Verification items for the finished model (mm, model axes). A direction names the side the tool comes from. Give positions to 0.01 mm unless a question says otherwise; leave off trailing zeros. Write each loop counter-clockwise with the first axis right and the second up, starting at its lowest first coordinate (ties: lowest second). Pieces come first, ordered by that corner, then holes. Notation, with made-up numbers: M 51,-23.75 L 67,-23.75 A20 ccw 67,14.25 Z; hole C 56,66.5 d6. An arc over 180 degrees is marked long. Answer as a JSON object with one key per item and string values.
```python
from build123d import *

# Parameters (mm, degrees)
CROQUIS1_W              = 100
CROQUIS1_H              = 100
SALIENTE_EXTRUIR1_DEPTH = 5
CHAFL_N1_SIZE2          = 2.886751346
CHAFL_N1_SIZE           = 5
CORTAR_EXTRUIR1_REACH   = 72.887
CROQUIS2_W              = 25
CROQUIS2_H              = 35


with BuildPart() as part:
    # Croquis1 → Saliente-Extruir1 (new body)
    with BuildSketch(Plane(origin=(0, 0, 0), x_dir=(1, 0, 0), z_dir=(0, 1, 0))):
        Rectangle(CROQUIS1_W, CROQUIS1_H)
    extrude(amount=SALIENTE_EXTRUIR1_DEPTH)

    # Chaflán1
    chafl_n1_edges = [part.edges().sort_by_distance(p)[0] for p in [
        (0, 5, 50),
    ]]
    chafl_n1_side = [part.faces().sort_by_distance(p)[0] for p in [
        (0, 4.942264973, 50),
    ]]
    chamfer(chafl_n1_edges, length=CHAFL_N1_SIZE - 0.0001, length2=CHAFL_N1_SIZE2 - 0.0001, reference=chafl_n1_side[0])  # a hair under: the kernel refuses the full size

    # Croquis2 → Cortar-Extruir1 (cut, up to next)
    with BuildSketch(Plane(origin=(0, 5, 0), x_dir=(1, 0, 0), z_dir=(0, 1, 0)), mode=Mode.PRIVATE) as cortar_extruir1_sk1:
        with Locations((-37.5, 32.5)):
            Rectangle(CROQUIS2_W, CROQUIS2_H)
    cortar_extruir1_tool1 = extrude(cortar_extruir1_sk1.sketch, amount=-CORTAR_EXTRUIR1_REACH, mode=Mode.PRIVATE) & part.part
    # Croquis2 → Cortar-Extruir1 (cut, up to next)
    with BuildSketch(Plane(origin=(0, 5, 0), x_dir=(1, 0, 0), z_dir=(0, 1, 0)), mode=Mode.PRIVATE) as cortar_extruir1_sk2:
        with Locations((37.5, 32.5)):
            Rectangle(CROQUIS2_W, CROQUIS2_H)
    cortar_extruir1_tool2 = extrude(cortar_extruir1_sk2.sketch, amount=-CORTAR_EXTRUIR1_REACH, mode=Mode.PRIVATE) & part.part
    add(cortar_extruir1_tool1.solids().sort_by_distance((-37.5, 5, -32.5))[0], mode=Mode.SUBTRACT)
    add(cortar_extruir1_tool2.solids().sort_by_distance((37.5, 5, -32.5))[0], mode=Mode.SUBTRACT)


solid = part.part
```
1) Thickness scan on L1, parallel to X at y = 0.25, z = -31.5; L2, parallel to Z at x = -44.5, y = 4.3; L3, parallel to Z at x = 15, y = 3.05. Record the ranges inside material, lowest first.
Completed:
{"L1": "x = -25 to 25", "L2": "z = -15 to 47.52", "L3": "z = -50 to 48.24"}
2) Section check C-C on z = -40.5. Record the boundary of the cut face in (x, y), and give its area (3 significant figures).
Completed:
{"outline": "M -25,0 L 25,0 L 25,5 L -25,5 Z", "area": "250 mm2"}
3) Access from +Z, -Z, +X, -X, +Y, -Y to the whole of each face (thin tool, end or side, straight path). Record for faces 1 (the face through (-25, 3, -32)), 2 (the face through (37, 3, -15)), 3 (the face through (-1, 0, 10)).
Completed:
{"face 1": "-Z, -X, +Y, -Y", "face 2": "-Z, +X, +Y, -Y", "face 3": "+Z, -Z, +X, -X, -Y"}
4) Section check B-B on y = 2.45. Record the boundary of the cut face in (x, z).
Completed:
{"outline": "M -50,-15 L -25,-15 L -25,-50 L 25,-50 L 25,-15 L 50,-15 L 50,48.59 L -50,48.59 Z"}
5) Go/stop test with flat-tipped pins: pin 1 (2 mm diameter, centred on x = 29.5, y = 4, fed in from +Z); pin 2 (1.5 mm diameter, centred on x = 33.5, y = 2.5, fed in from -Z). Record where each tip stops, or that it passes through.
Completed:
{"pin 1": "stops at z = 48.27", "pin 2": "stops at z = -15"}
